```python
from build123d import *

# Parameters (mm, degrees)
F0_R     = 16.4465
F1_DEPTH = 101.6
F4_DEPTH = 101.601
F5_D     = 3.4544
F5_DEPTH = 16.4475
F6_D     = 3.4544
F6_DEPTH = 16.4475001


with BuildPart() as f1:
    # F0 (on Right) → F1 (new body)
    with BuildSketch(Plane.YZ):
        Circle(F0_R)
    extrude(amount=F1_DEPTH)

    # F2 (on face) → F4 (cut, through all)
    with BuildSketch(Plane.YZ.offset(101.6)):
        with BuildLine():
            ThreePointArc((13.9065, 0), (0, 13.9065), (-13.9065, 0))
            ThreePointArc((-13.9065, 0), (0, -13.9065), (13.9065, 0))
        make_face()
    extrude(amount=-F4_DEPTH, mode=Mode.SUBTRACT)

    # F5 (through all, one way)
    with BuildSketch(Plane.XZ):
        with Locations((71.1848556182, 0)):
            Circle(F5_D / 2)
    extrude(amount=-F5_DEPTH, mode=Mode.SUBTRACT)

    # F6 (through all, one way)
    with BuildSketch(Plane.XZ):
        with Locations((55.9448556182, 0)):
            Circle(F6_D / 2)
    extrude(amount=-F6_DEPTH, mode=Mode.SUBTRACT)


solid = f1.part
```
Geometry: final body of the model. Coordinates: model frame, mm. Coordinates: 2 decimals unless noted, no trailing zeros. Order: outer loops, then holes, each group sorted by start corner. A loop starts at its lowest first (then second) coordinate and runs counter-clockwise, first axis right, second up. Notation, with made-up numbers: (74.5, 86.5) -> (100.5, 86.5) arc R15 ccw to (100.5, 107.5) -> close; hole circle Ø3 at (53, -33). An arc over 180 degrees is marked (long way). Write item = value, one per line.
(1) Cut plane B-B on z = 0. Return loops of the section in (x, y), plus the area to 3 significant figures.
Solved:
outline = (0, -16.45) -> (101.6, -16.45) -> (101.6, -13.91) -> (0, -13.91) -> close; (0, 13.91) -> (54.22, 13.91) -> (54.22, 16.45) -> (0, 16.45) -> close; (57.67, 13.91) -> (69.46, 13.91) -> (69.46, 16.45) -> (57.67, 16.45) -> close; (72.91, 13.91) -> (101.6, 13.91) -> (101.6, 16.45) -> (72.91, 16.45) -> close
area = 499 mm²
(2) Pin query (flat end, axial travel): pin 1 Ø6 at (x, z) = (76.5, -7.5) entering from -Y; pin 2 Ø12 at (x, y) = (21, 9) entering from -Z; pin 3 Ø5 at (x, y) = (31, 12.5) entering from -Z; pin 4 Ø5 at (y, z) = (-6.5, 6.5) entering from +X. Return the tip coordinate at first contact, or that it passes through.
Solved:
pin_1 = -15.82
pin_2 = -16.17
pin_3 = -13.06
pin_4 = through
(3) Cut plane C-C on z = 7. Return loops of the section in (x, y), plus the area to 3 significant figures.
Solved:
outline = (0, -14.88) -> (101.6, -14.88) -> (101.6, -12.02) -> (0, -12.02) -> close; (0, 12.02) -> (101.6, 12.02) -> (101.6, 14.88) -> (0, 14.88) -> close
area = 582 mm²
(4) Cut plane D-D on x = 28. Return loops of the section in (y, z).
Solved:
outline = circle Ø32.89 at (0, 0); hole circle Ø27.81 at (0, 0)
(5) Pull-direction query (X, two-part tool) for faces 1 (the cylindrical face through (51.511, 3.015, 13.576)), 2 (the cylindrical face through (69.46, 15.1, 0.08)), 3 (the cylindrical face through (54.22, 15.1, 0.08)), 4 (the flat face through (101.6, -12.3, 7.4)); classes: pulls with the +X half, pulls with the -X half, needs draft (parallel to the pull), parting line crosses it, or undercut.
Solved:
face_1 = needs draft
face_2 = undercut
face_3 = undercut
face_4 = pulls with the +X half
(6) Line query: line 1 (X direction, y = 15, z = 0); line 2 (Y direction, x = 25, z = -0.5); line 3 (Z direction, x = 35, y = 0). Output: solid intervals per line, ascending.
Solved:
line_1 = 0 to 54.22, 57.67 to 69.46, 72.91 to 101.6
line_2 = -16.44 to -13.9, 13.9 to 16.44
line_3 = -16.45 to -13.91, 13.91 to 16.45
(7) Cut plane A-A on y = 0. Return loops of the section in (x, z).
Solved:
outline = (0, -16.45) -> (101.6, -16.45) -> (101.6, -13.91) -> (0, -13.91) -> close; (0, 13.91) -> (101.6, 13.91) -> (101.6, 16.45) -> (0, 16.45) -> close
